Here's how the part is built. I have some questions about the finished solid (model axes, mm). A direction names the side the tool comes from. Coordinates: 2 decimals unless noted, no trailing zeros. Loops run counter-clockwise (first coordinate to the right, second up) from the corner with the lowest first, then second, coordinate; pieces in that order, holes last. Notation, with made-up numbers: (75.5, 68.5) -> (117.5, 68.5) arc R22 cw to (117.5, 93.5) -> close; hole circle Ø8 at (55, 51.25). An arc over 180 degrees is marked (long way). Answer as a JSON object with one key per item and string values. Group by question number.
Q1. Thinking about a two-plate mould opening in Y: for faces 3 (the cylindrical face through (-158.346, 24.9, -17.986)), 4 (the flat face through (-158, 20, -9)), 5 (the cylindrical face through (-153.577, 26.402, -13.766)), which applies, released by +Y, released by -Y, zero draft, split by the parting line, or undercut?
Q2. I'm going to push flat-ended pins straight in: pin 1 (2 mm diameter, centred on y = 22.5, z = -11, fed in from -X); pin 2 (3 mm diameter, centred on x = -159.3, y = 24.6, fed in from +Z). Where does each tip first touch, or does it pass through?
Q3. I want a section at C-C on z = -15.25. Write out the boundary of the cut face in (x, y), then the cut area to 3 significant figures.
Q4. I want a section at A-A on x = -159.3. Write out the boundary of the cut face in (y, z).
Q5. On a 3-axis mill with a long thin cutter (end or side, diameter ignored), from which of +Z, -Z, +X, -X, +Y, -Y can I reach the whole of each face in a straight line? I mean faces 1 (the flat face through (-159, 23, -19)), 2 (the cylindrical face through (-162.5, 22.2, -13.2)). Say none if no direction works.
Q6. I need wall thicknesses on line 1 (Y direction, x = -159.3, z = -13); line 2 (Y direction, x = -159.3, z = -17.6); line 3 (Z direction, x = -159.75, y = 25.75). Which ranges of each line are inside material? Lowest first, please.
Q7. I want a section at B-B on y = 24.6. Write out the boundary of the cut face in (x, z).
```python
from build123d import *

# Parameters (mm, degrees)
CHAMFER_SIZE    = 0.6
CHAMFER001_SIZE = 0.6


with BuildPart() as part:
    # Sketch010 → Revolution001 (revolve)
    with BuildSketch(Plane.XZ):
        Polygon((1, -8), (4, -8), (4, 0), (6, 0), (6, -10), (1, -10), align=None)
    revolve(axis=Axis((0, 0, 0), (0, 0, 1)))

    # Chamfer
    chamfer_edges = [part.edges().sort_by_distance(p)[0] for p in [
        (-6, 0, -10),
    ]]
    chamfer(chamfer_edges, length=CHAMFER_SIZE)

    # Chamfer001
    chamfer001_edges = [part.edges().sort_by_distance(p)[0] for p in [
        (-4, 0, 0),
    ]]
    chamfer(chamfer001_edges, length=CHAMFER001_SIZE)


with BuildPart() as part_1:
    # Body007 placement: moved
    add(part.part.moved(Location((-159.3, 24.6, -9))))


solid = part_1.part
```
Result set:
{
 "1": {"face 3": "undercut", "face 4": "zero draft", "face 5": "split by the parting line"},
 "2": {"pin 1": "stops at x = -165.2", "pin 2": "stops at z = -17"},
 "3": {"outline": "circle Ø12 at (-159.3, 24.6); hole circle Ø8 at (-159.3, 24.6)", "area": "62.8 mm²"},
 "4": {"outline": "(18.6, -18.4) -> (19.2, -19) -> (23.6, -19) -> (23.6, -17) -> (20.6, -17) -> (20.6, -9.6) -> (20, -9) -> (18.6, -9) -> close; (25.6, -19) -> (30, -19) -> (30.6, -18.4) -> (30.6, -9) -> (29.2, -9) -> (28.6, -9.6) -> (28.6, -17) -> (25.6, -17) -> close"},
 "5": {"face 1": "-Z, +X, -X, +Y, -Y", "face 2": "+Z"},
 "6": {"line 1": "y = 18.6 to 20.6, 28.6 to 30.6", "line 2": "y = 18.6 to 23.6, 25.6 to 30.6", "line 3": "z = -19 to -17"},
 "7": {"outline": "(-165.3, -18.4) -> (-164.7, -19) -> (-160.3, -19) -> (-160.3, -17) -> (-163.3, -17) -> (-163.3, -9.6) -> (-163.9, -9) -> (-165.3, -9) -> close; (-158.3, -19) -> (-153.9, -19) -> (-153.3, -18.4) -> (-153.3, -9) -> (-154.7, -9) -> (-155.3, -9.6) -> (-155.3, -17) -> (-158.3, -17) -> close"}
}
